```python
from build123d import *

# Parameters (mm, degrees)
F0_W     = 160
F0_H     = 8
F0_H_2   = 4
F0_H_3   = 74
F1_DEPTH = 12
F2_DEPTH = 20


with BuildPart() as f1:
    # F0 (on Front) → F1 (new body)
    with BuildSketch(Plane.XZ):
        with Locations((0, 41)):
            Rectangle(F0_W, F0_H)
        with Locations((0, 35)):
            Rectangle(F0_W, F0_H_2)
        with Locations((0, -4)):
            Rectangle(F0_W, F0_H_3)
        with Locations((0, -43)):
            Rectangle(F0_W, F0_H_2)
    extrude(amount=F1_DEPTH)

    # F0 (on Front) → F2 (join)
    with BuildSketch(Plane.XZ):
        with Locations((0, 41)):
            Rectangle(F0_W, F0_H)
        with Locations((0, -4)):
            Rectangle(F0_W, F0_H_3)
    extrude(amount=F2_DEPTH)


solid = f1.part
```
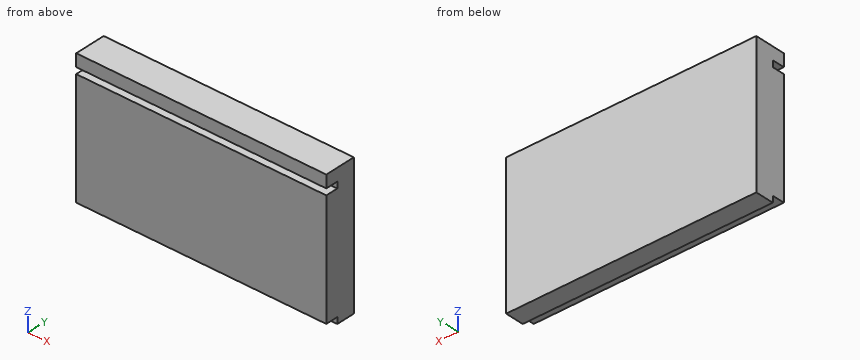
Here's how the part is built. I have some questions about the finished solid (model axes, mm). Coordinates: 2 decimals unless noted, no trailing zeros. Loops run counter-clockwise (first coordinate to the right, second up) from the corner with the lowest first, then second, coordinate; pieces in that order, holes last. Notation, with made-up numbers: (88.25, 67.5) - (92.25, 67.5) arc R10 cw to (92.25, 77.5) - close; hole circle Ø9 at (1.25, 56.25). An arc over 180 degrees is marked (long way). Answer as CSV lines item,"result".
Q1. If we section it at B-B, the plane x = 43: Write out the boundary of the cut face in (y, z), and give its area (3 significant figures).
Response:
outline,"(-20, -41) - (-12, -41) - (-12, -45) - (0, -45) - (0, 45) - (-20, 45) - (-20, 37) - (-12, 37) - (-12, 33) - (-20, 33) - close"
area,"1,740 mm2"
Q2. For pin 1 (2 mm diameter, centred on x = -61.5, y = -17, fed in from -Z); pin 2 (2 mm diameter, centred on x = -12, z = 35.5, fed in from -Y); pin 3 (8 mm diameter, centred on x = 20, z = -1, fed in from +Y), each with a flat end and sliding along its axis, tell me the tip position at first contact or that it passes through.
Response:
pin 1,"z = -41"
pin 2,"y = -12"
pin 3,"y = 0"
Q3. If we section it at A-A, the plane y = -18: Write out the boundary of the cut face in (x, z).
Response:
outline,"(-80, -41) - (80, -41) - (80, 33) - (-80, 33) - close; (-80, 37) - (80, 37) - (80, 45) - (-80, 45) - close"
Q4. If I drill on L1, parallel to Z at x = 42.5, y = -14.5, over which ranges is the centre line in solid material (lowest first)? Write a range as [from, to].
Response:
L1,"[-41, 33], [37, 45]"
Q5. If we section it at C-C, the plane z = 34.5: Write out the boundary of the cut face in (x, y), and give its area (3 significant figures).
Response:
outline,"(-80, -12) - (80, -12) - (80, 0) - (-80, 0) - close"
area,"1,920 mm2"
